```python
from build123d import *

# Parameters (mm, degrees)
F0_R     = 6.9
F0_R_2   = 1.5
F1_DEPTH = 10
F2_R     = 4
F3_DEPTH = 4
F4_SIZE  = 0.5


with BuildPart() as f1:
    # F0 (on Top) → F1 (new body)
    with BuildSketch(Plane.XY):
        Circle(F0_R)
        Circle(F0_R_2, mode=Mode.SUBTRACT)
    extrude(amount=F1_DEPTH)

    # F2 (on face) → F3 (cut)
    with BuildSketch(Plane.XY.offset(10)):
        Circle(F2_R)
    extrude(amount=-F3_DEPTH, mode=Mode.SUBTRACT)

    # F4
    f4_edges = [f1.edges().sort_by_distance(p)[0] for p in [
        (-1.5, 0, 6),
    ]]
    chamfer(f4_edges, length=F4_SIZE)


solid = f1.part
```
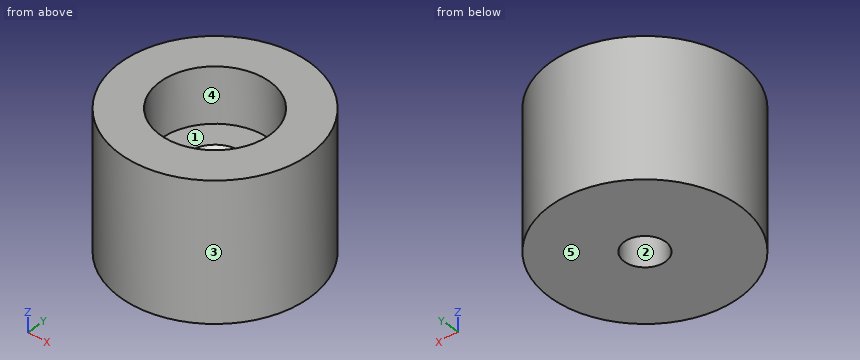
CAD build for the part. Positions are in the model's coordinates, mm. Face numbers are marked on the shaded views. A direction names the side the tool comes from. Round coordinates to 2 decimals unless told otherwise and drop trailing zeros. Loops run counter-clockwise (first coordinate to the right, second up) from the corner with the lowest first, then second, coordinate; pieces in that order, holes last. Notation, with made-up numbers: (-34, 27) - (7, 27) arc R28 ccw to (7, 62) - close; hole circle Ø7 at (-37, 88). An arc over 180 degrees is marked (long way). Return JSON: item names as keys, results as strings. Group by question number.
Q1. Band-saw the part on A-A on y = 0. Give the cut face in (x, z), plus the area to 4 significant figures.
Q2. Flat gauge pins, fed straight in: pin 1 Ø2.5 at (x, y) = (-0.5, -1) entering from +Z; pin 2 Ø1 at (x, z) = (4, 3) entering from -Y; pin 3 Ø1.5 at (x, z) = (-4.5, 5) entering from +Y; pin 4 Ø2.5 at (x, y) = (0, 0) entering from -Z. Where does each tip first touch, or does it go through?
Q3. Tool access for the marked faces 1 and 2: list every direction of +Z, -Z, +X, -X, +Y, -Y with a clear straight run to the whole face (end or side of a thin tool).
Q4. Two-plate mould, pull along X, no slides. Class the marked faces 3, 4 and 5: +X half, -X half, draft (parallel to the pull), parting line (faces both ways), or undercut.
Q5. Drill centre lines: line 1 along Y through (x, z) = (0, 6.8); line 2 along Y through (x, z) = (0, 2.7); line 3 along X through (y, z) = (1.5, 5.75). Where is each one in solid material? Low to high. Write a range as [from, to].
Q6. Band-saw the part on C-C on z = 3. Give the cut face in (x, y), plus the area to 3 significant figures.
Q7. Band-saw the part on D-D on y = -2.25. Give the cut face in (x, z), plus the area to 3 significant figures.
Solutions:
{
 "1": {"outline": "(-6.9, 0) - (-1.5, 0) - (-1.5, 5.5) - (-2, 6) - (-4, 6) - (-4, 10) - (-6.9, 10) - close; (1.5, 0) - (6.9, 0) - (6.9, 10) - (4, 10) - (4, 6) - (2, 6) - (1.5, 5.5) - close", "area": "87.75 mm^2"},
 "2": {"pin 1": "stops at z = 6", "pin 2": "stops at y = -5.95", "pin 3": "stops at y = 5.79", "pin 4": "passes through"},
 "3": {"face 1": "+Z", "face 2": "+Z, -Z"},
 "4": {"face 3": "parting line", "face 4": "undercut", "face 5": "draft"},
 "5": {"line 1": "y = [-6.9, -4], [4, 6.9]", "line 2": "y = [-6.9, -1.5], [1.5, 6.9]", "line 3": "x = [-6.73, -0.9], [0.9, 6.73]"},
 "6": {"outline": "circle Ø13.8 at (0, 0); hole circle Ø3 at (0, 0)", "area": "143 mm^2"},
 "7": {"outline": "(-6.52, 0) - (6.52, 0) - (6.52, 10) - (3.31, 10) - (3.31, 6) - (-3.31, 6) - (-3.31, 10) - (-6.52, 10) - close", "area": "104 mm^2"}
}
